Build history of the part. All positions in model axes, mm. A direction names the side the tool comes from. Round coordinates to 2 decimals unless told otherwise and drop trailing zeros. Loops run counter-clockwise (first coordinate to the right, second up) from the corner with the lowest first, then second, coordinate; pieces in that order, holes last. Notation, with made-up numbers: (-38, -16) - (-19, -16) arc R16 cw to (-19, -6) - close; hole circle Ø5 at (-7, 10.5). An arc over 180 degrees is marked (long way). Use one line per item in the form item = value. Start each with the question number.
Q1. Drill centre lines: line 1 (X direction, y = -17.95, z = 97.2); line 2 (Y direction, x = -18.5, z = 87.5); line 3 (Z direction, x = -2.5, y = 17.5). Where is each one in solid material? Low to high.
Q2. 3-axis set-ups, long thin cutter, end or side, ignore diameter. For faces 5 (the face through (-10, 11, 94.7)), 6 (the face through (-18, 18, 99.7)): which of +Z, -Z, +X, -X, +Y, -Y reach the whole face in a straight line?
Q3. Saw through at B-B (z = 97.2). Give the cut face in (x, y), then the cut area to 3 significant figures.
Q4. Saw through at D-D (x = -16). Give the cut face in (y, z).
Q5. Pin check, flat tips, straight feed: pin 1 (1.5 mm diameter, centred on x = -4, y = 8, fed in from +Z); pin 2 (2.5 mm diameter, centred on x = -34.5, z = 97.2, fed in from -Y). Stop position of each tip, or through.
Q6. Saw through at C-C (x = -34.5). Give the cut face in (y, z), then the cut area to 3 significant figures.
Q7. Mould opens along X. For faces 1 (the face through (-5.22, 0.58, 88.72)), 2 (the face through (-33.77, -18.35, 98.61)), 3 (the face through (-6, 5, 82.912)), 4 (the face through (0, 0, 89)) say: released by +X, released by -X, zero draft, split by the parting line, or undercut.
Q8. Saw through at A-A (y = 0). Give the cut face in (x, z).
Autodesk Inventor part; units mm, degrees
ref_plane "YZ Plane" through (0, 0, 0) normal (1, 0, 0) x (0, 1, 0)
ref_plane "XZ Plane" through (0, 0, 0) normal (0, 1, 0) x (-1, 0, 0)
ref_plane "XY Plane" through (0, 0, 0) normal (0, 0, 1) x (1, 0, 0)
sketch "Sketch2" plane through (0, 0, 0) normal (1, 0, 0) x (0, 1, 0)
  circle A0 centre (0, 0) radius 13.2937
  line L0 (-16, -18.5) -> (16, -18.5)
  line L1 (16, -18.5) -> (16, 18.5)
  line L2 (16, 18.5) -> (-16, 18.5)
  line L3 (-16, 18.5) -> (-16, -18.5)
  line L4 (-16, -18.5) -> (16, 18.5) construction
  line L5 (16, -18.5) -> (-16, 18.5) construction
  dimension "d9" = 26.5875
  dimension "d10" = 32
  dimension "d11" = 37
extrude "Extrusion2" add sketch "Sketch2" along normal blind 76.2
sketch "Sketch3" plane through (0, -16, -18.5) normal (0, 0, -1) x (-1, 0, 0)
  line L0 (0, 0) -> (0, 32)
  circle A0 centre (18.5, 16) radius 13.2937
  line L1 (0, 32) -> (0, 0)
  line L2 (0, 0) -> (37, 0)
  line L3 (37, 0) -> (37, 32)
  line L4 (37, 32) -> (0, 32)
  line L5 (0, 32) -> (37, 0) construction
  line L6 (0, 0) -> (37, 32) construction
  point P0 (0, 16)
  dimension "d14" = 26.5875
  dimension "d15" = 32
  dimension "d16" = 37
extrude "Extrusion3" add sketch "Sketch3" against normal blind 113.2
sketch "Sketch4" plane through (76.2, -16, -18.5) normal (0, 0, -1) x (-1, 0, 0)
  circle A0 centre (94.7, 16) radius 13.2937
  point P0 (76.2, 16)
extrude "Extrusion4" add sketch "Sketch4" against normal blind 37
sketch "Sketch5" plane through (76.2, 16, 18.5) normal (0, 1, 0) x (1, 0, 0)
  line L0 (-113.2, 37) -> (0, 37)
  line L1 (-113.2, 37) -> (-113.2, -76.2)
  line L2 (-113.2, 37) -> (-100.1185, 50.0815)
  line L3 (-113.2, 37) -> (-94.7, 37) construction
  line L4 (-113.2, 37) -> (-126.2815, 23.9185)
  line L5 (-113.2, 37) -> (-94.7, 37) construction
  line L6 (-100.1185, 50.0815) -> (-154.0001, 103.963)
  line L7 (-126.2815, 23.9185) -> (-180.163, 77.8001)
  line L8 (-126.2815, 23.9185) -> (-50.0815, 23.9185) construction
  line L9 (-154.0001, 103.963) -> (-180.163, 77.8001)
  line L10 (-100.1185, 50.0815) -> (-87.037, 37)
  line L11 (-126.2815, 23.9185) -> (-113.2, 10.837)
  point P0 (-76.2, 18.5)
  dimension "d21" = 18.5
  dimension "d22" = 45
  dimension "d23" = 18.5
  dimension "d24" = 135
  dimension "d25" = 76.2
  dimension "d26" = 76.2
  dimension "d27" = 135
extrude "Extrusion5" add sketch "Sketch5" against normal blind 32
sketch "Sketch7" plane through (-77.8001, -16, -85.463) normal (-0.7071, 0, -0.7071) x (-0.7071, 0, 0.7071)
  line L0 (37, 0) -> (37, 32)
  line L1 (37, 32) -> (0, 32)
  line L2 (0, 32) -> (0, 0)
  line L3 (0, 0) -> (37, 0)
  circle A0 centre (18.5, 16) radius 13.2937
  point P0 (5.4185, 16)
  point P1 (37, 16)
extrude "Extrusion6" cut sketch "Sketch7" against normal blind 101.6 contours A0
sketch "Sketch8" plane through (76.2, 16, 18.5) normal (0, 1, 0) x (1, 0, 0)
  line L0 (-76.2, 0) -> (0, 0)
  line L1 (-87.037, 37) -> (0, 37)
  line L2 (-87.037, 37) -> (-154.0001, 103.963)
  line L3 (-180.163, 77.8001) -> (-113.2, 10.837)
  line L4 (-113.2, 10.837) -> (-113.2, -76.2)
  line L5 (-76.2, 0) -> (-76.2, -76.2)
  line L6 (0, 37) -> (5, 37)
  line L7 (5, 37) -> (5, 0)
  line L8 (5, 0) -> (0, 0)
  line L9 (0, 0) -> (0, 37)
  line L10 (-113.2, -76.2) -> (-76.2, -76.2)
  line L11 (-76.2, -76.2) -> (-76.2, -81.2)
  line L12 (-76.2, -81.2) -> (-113.2, -81.2)
  line L13 (-113.2, -81.2) -> (-113.2, -76.2)
  line L14 (-180.163, 77.8001) -> (-183.6985, 81.3356)
  line L15 (-183.6985, 81.3356) -> (-157.5356, 107.4985)
  line L16 (-157.5356, 107.4985) -> (-154.0001, 103.963)
  point P0 (-76.2, 18.5)
  dimension "d32" = 5
  dimension "d33" = 5
  dimension "d34" = 5
  dimension "d35" = 90
extrude "Extrusion7" add sketch "Sketch8" along normal blind 4.7752
sketch "Sketch9" plane through (76.2, -16, -18.5) normal (0, -1, 0) x (1, 0, 0)
  line L0 (-87.037, 0) -> (0, 0)
  line L1 (-76.2, 37) -> (0, 37)
  line L2 (-76.2, 37) -> (-76.2, 113.2)
  line L3 (-113.2, 26.163) -> (-113.2, 113.2)
  line L4 (-113.2, 26.163) -> (-180.163, -40.8001)
  line L5 (-154.0001, -66.963) -> (-87.037, 0)
  line L6 (-76.2, 118.2) -> (-76.2, 37)
  line L7 (-113.2, 113.2) -> (-76.2, 113.2)
  line L8 (-76.2, 113.2) -> (-76.2, 118.2)
  line L9 (-76.2, 118.2) -> (-113.2, 118.2)
  line L10 (-113.2, 118.2) -> (-113.2, 113.2)
  line L11 (-76.2, 37) -> (5, 37)
  line L12 (0, 0) -> (5, 0)
  line L13 (5, 0) -> (5, 37)
  line L14 (5, 37) -> (0, 37)
  line L15 (0, 37) -> (0, 0)
  line L16 (-183.6985, -44.3356) -> (-113.2, 26.163)
  line L17 (-180.163, -40.8001) -> (-183.6985, -44.3356)
  line L18 (-183.6985, -44.3356) -> (-157.5356, -70.4985)
  line L19 (-157.5356, -70.4985) -> (-154.0001, -66.963)
  point P0 (-76.2, 18.5)
extrude "Extrusion8" add sketch "Sketch9" along normal blind 4.7752
sketch "Sketch10" plane through (76.2, 20.7752, 18.5) normal (0, 1, 0) x (1, 0, 0)
  circle A0 centre (2.5, 34.5) radius 1.5875
  circle A1 centre (2.5, 2.5) radius 1.5875
  line L0 (0, 37) -> (0, 0)
  line L1 (0, 0) -> (5, 0)
  line L2 (5, 37) -> (5, 0)
  line L3 (0, 37) -> (5, 37)
  point P0 (-76.2, 18.5)
  point P1 (0, 18.5)
extrude "Extrusion9" cut sketch "Sketch10" against normal blind 279.4 contours A0 | A1
sketch "Sketch11" plane through (76.2, 20.7752, 18.5) normal (0, 1, 0) x (1, 0, 0)
  circle A0 centre (-78.7, -78.7) radius 1.5875
  circle A1 centre (-110.7, -78.7) radius 1.5875
  line L0 (-76.2, -76.2) -> (-113.2, -76.2)
  line L1 (-113.2, -76.2) -> (-113.2, -81.2)
  line L2 (-76.2, -81.2) -> (-113.2, -81.2)
  line L3 (-76.2, -76.2) -> (-76.2, -81.2)
  circle A2 centre (-157.5356, 103.963) radius 1.5875
  circle A3 centre (-180.163, 81.3356) radius 1.5875
  line L4 (-157.5356, 107.4985) -> (-183.6985, 81.3356)
  line L5 (-183.6985, 81.3356) -> (-180.163, 77.8001)
  line L6 (-154.0001, 103.963) -> (-180.163, 77.8001)
  line L7 (-157.5356, 107.4985) -> (-154.0001, 103.963)
  point P0 (-76.2, 18.5)
  point P1 (-94.7, -76.2)
  point P2 (-170.6171, 94.4171)
extrude "Extrusion10" cut sketch "Sketch11" against normal blind 279.4 contours A0 | A1 | A2 | A3
sketch "Sketch12" plane through (76.2, 20.7752, 18.5) normal (0, 1, 0) x (1, 0, 0)
  circle A0 centre (-157.5356, 103.963) radius 1.5875
  circle A1 centre (-180.163, 81.3356) radius 1.5875
  circle A2 centre (2.5, 2.5) radius 1.5875
  circle A3 centre (2.5, 34.5) radius 1.5875
  line L0 (-204.7971, 116.7224) -> (14.3752, 116.7224)
  line L1 (14.3752, 116.7224) -> (14.3752, -64.4123)
  line L2 (14.3752, -64.4123) -> (-204.7971, -64.4123)
  line L3 (-204.7971, -64.4123) -> (-204.7971, 116.7224)
  point P0 (-76.2, 18.5)
extrude "Extrusion11" cut sketch "Sketch12" against normal blind 76.2
properties part number "testPrintBracket"
Report:
q1.line_1 = -37 to -36.09, -32.91 to -4.09, -0.91 to 0
q1.line_2 = -20.78 to -13.29, 13.29 to 20.78
q1.line_3 = 82.91 to 95.61, 98.79 to 99.7
q2.face_5 = +Z, +X, -X
q2.face_6 = +Z, +X, -X, +Y, -Y
q3.outline = (-37, -20.78) - (-36.09, -20.78) - (-36.09, -16) - (-37, -16) - close; (-37, 16) - (-36.09, 16) - (-36.09, 20.78) - (-37, 20.78) - close; (-32.91, -20.78) - (-4.09, -20.78) - (-4.09, -16) - (-32.91, -16) - close; (-32.91, 16) - (-4.09, 16) - (-4.09, 20.78) - (-32.91, 20.78) - close; (-0.91, -20.78) - (0, -20.78) - (0, -16) - (-0.91, -16) - close; (-0.91, 16) - (0, 16) - (0, 20.78) - (-0.91, 20.78) - close
q3.area = 293 mm²
q4.outline = (-20.78, 82.91) - (-13.06, 82.91) - (-13.06, 94.7) - (-16, 94.7) - (-16, 99.7) - (-20.78, 99.7) - close; (13.06, 82.91) - (20.78, 82.91) - (20.78, 99.7) - (16, 99.7) - (16, 94.7) - (13.06, 94.7) - close
q5.pin_1 = 94.7
q5.pin_2 = through
q6.outline = (-20.78, 82.91) - (20.78, 82.91) - (20.78, 95.61) - (16, 95.61) - (16, 94.7) - (-16, 94.7) - (-16, 95.61) - (-20.78, 95.61) - close; (-20.78, 98.79) - (-16, 98.79) - (-16, 99.7) - (-20.78, 99.7) - close; (16, 98.79) - (20.78, 98.79) - (20.78, 99.7) - (16, 99.7) - close
q6.area = 507 mm²
q7.face_1 = undercut
q7.face_2 = undercut
q7.face_3 = zero draft
q7.face_4 = released by +X
q8.outline = (-37, 82.91) - (-31.79, 82.91) - (-31.79, 94.7) - (-37, 94.7) - close; (-5.21, 82.91) - (0, 82.91) - (0, 94.7) - (-5.21, 94.7) - close
